```python
from build123d import *

# Parameters (mm, degrees)
F0_R     = 25.4
F0_R_2   = 12.7
F1_DEPTH = 6.35
F2_DEPTH = 3.175


with BuildPart() as f1:
    # F0 (on Front) → F1 (new body)
    with BuildSketch(Plane.XZ):
        Polygon((0, 38.1), (0, 0), (25.4, 0), (76.2, 0), (139.7, 0), (139.7, 50.8), (107.95, 101.6), (0, 101.6), (0, 63.5), align=None)
        with Locations((76.2, 38.1)):
            Circle(F0_R, mode=Mode.SUBTRACT)
        with Locations((25.4, 63.5)):
            Circle(F0_R_2, mode=Mode.SUBTRACT)
        with Locations((76.2, 38.1)):
            Circle(F0_R)
        with Locations((76.2, 38.1)):
            Circle(F0_R_2, mode=Mode.SUBTRACT)
    extrude(amount=-F1_DEPTH)

    # F0 (on Front) → F2 (join)
    with BuildSketch(Plane.XZ):
        with Locations((76.2, 38.1)):
            Circle(F0_R)
        with Locations((76.2, 38.1)):
            Circle(F0_R_2, mode=Mode.SUBTRACT)
    extrude(amount=F2_DEPTH)


solid = f1.part
```
Geometry: final body of the model. Coordinates: model frame, mm. Round coordinates to 2 decimals unless told otherwise and drop trailing zeros. Order: outer loops, then holes, each group sorted by start corner. A loop starts at its lowest first (then second) coordinate and runs counter-clockwise, first axis right, second up. Notation, with made-up numbers: (-37, 9.5) - (-14, 9.5) arc R21 ccw to (-14, 14.5) - close; hole circle Ø8 at (77, 7.25). An arc over 180 degrees is marked (long way). Write item = value, one per line. Start each with the question number.
Q1. Ray query, line 1 (Z direction, x = 25.4, y = 4.75); line 2 (Y direction, x = 127.5, z = 26.5); line 3 (X direction, y = 5, z = 74). Return the intervals inside material, ascending. Write a range as from..to.
Q2. Cut plane B-B on z = 38.1. Return the cut outline in (x, y) (3 decimals), and give its area (3 significant figures).
Q3. Pull-direction query (Z, two-part tool) for faces 1 (the cylindrical face through (99.663, -1.565, 28.372)), 2 (the flat face through (139.7, 3, 25)), 3 (the cylindrical face through (12.712, 3.131, 64.058)); classes: +Z half, -Z half, draft (parallel to the pull), parting line (faces both ways), or undercut.
Q4. Cut plane C-C on y = 1.75. Return the cut outline in (x, z), and give its area (3 significant figures).
Q5. Cut plane A-A on x = 25.4. Return the cut outline in (y, z).
Q6. Cut plane D-D on x = 76.2. Return the cut outline in (y, z) (3 decimals), and give its area (3 significant figures).
Q7. Pin query (flat end, axial travel): pin 1 (3 mm diameter, centred on y = 0.5, z = 62, fed in from +X); pin 2 (20.5 mm diameter, centred on x = 25.4, z = 63.5, fed in from -Y); pin 3 (5 mm diameter, centred on x = 113.5, y = -1, fed in from +Z). Return the tip coordinate at first contact, or that it passes through.
Outcome:
q1.line_1 = 0..50.8, 76.2..101.6
q1.line_2 = 0..6.35
q1.line_3 = 0..18.26, 32.54..125.2
q2.outline = (0, 0) - (50.8, 0) - (50.8, -3.175) - (63.5, -3.175) - (63.5, 6.35) - (0, 6.35) - close; (88.9, -3.175) - (101.6, -3.175) - (101.6, 0) - (139.7, 0) - (139.7, 6.35) - (88.9, 6.35) - close
q2.area = 806 mm^2
q3.face_1 = parting line
q3.face_2 = draft
q3.face_3 = undercut
q4.outline = (0, 0) - (139.7, 0) - (139.7, 50.8) - (107.95, 101.6) - (0, 101.6) - close; hole circle Ø25.4 at (25.4, 63.5); hole circle Ø25.4 at (76.2, 38.1)
q4.area = 12,400 mm^2
q5.outline = (0, 0) - (6.35, 0) - (6.35, 50.8) - (0, 50.8) - close; (0, 76.2) - (6.35, 76.2) - (6.35, 101.6) - (0, 101.6) - close
q6.outline = (-3.175, 12.7) - (0, 12.7) - (0, 0) - (6.35, 0) - (6.35, 25.4) - (-3.175, 25.4) - close; (-3.175, 50.8) - (6.35, 50.8) - (6.35, 101.6) - (0, 101.6) - (0, 63.5) - (-3.175, 63.5) - close
q6.area = 565 mm^2
q7.pin_1 = 133.64
q7.pin_2 = through
q7.pin_3 = 96.39
